from build123d import *

# Parameters (mm, degrees)
EXTRUDE_4_OUTLINE_R  = 1.5999968
EXTRUDE_4_OUTLINE_W  = 44.323
EXTRUDE_4_OUTLINE_H  = 54.229
EXTRUDE_4_DEPTH      = 1.5
EXTRUDE_5_DEPTH      = 1.5
EXTRUDE_5_DEPTH_BACK = 13
SKETCH_3_W           = 44.323
SKETCH_3_H           = 54.229
SKETCH_5_R           = 1.27
SKETCH_5_W           = 14.0000228
SKETCH_5_H           = 32.0000376
EXTRUDE_6_DEPTH      = 13
EXTRUDE_8_DEPTH      = 1.5
EXTRUDE_8_DEPTH_BACK = 20
SKETCH_6_W           = 38.989
SKETCH_6_H           = 65.9999442
SKETCH_6_R           = 1.016
SKETCH_6_R_2         = 0.4572


# Read off the part's stored shape, not the designer's step: the extrude step
with BuildPart() as part:
    # Extrude 4 outline → Extrude 4 (new body)
    with BuildSketch(Plane.XY):
        with BuildLine():
            ThreePointArc((122.299984025, 9.019649552), (120.835516371, 12.55516818), (117.299994025, 14.019626857))
            Line((117.299994025, 14.019626857), (4.999990016, 14.019626857))
            ThreePointArc((4.999990016, 14.019626857), (1.464472156, 12.555172669), (1.1e-08, 9.019662248))
            Line((1.1e-08, 9.019662248), (1.1e-08, -60.980388257))
            ThreePointArc((1.1e-08, -60.980388257), (1.464467665, -64.515906885), (4.999990011, -65.980365562))
            Line((4.999990011, -65.980365562), (117.29999402, -65.980365562))
            ThreePointArc((117.29999402, -65.980365562), (120.835516369, -64.515906884), (122.299984025, -60.980388255))
            Line((122.299984025, -60.980388255), (122.299984025, 9.019649552))
        make_face()
        with Locations((4.999990011, -53.480365152)):
            Circle(EXTRUDE_4_OUTLINE_R, mode=Mode.SUBTRACT)
        with Locations((117.299994011, -53.480365152)):
            Circle(EXTRUDE_4_OUTLINE_R, mode=Mode.SUBTRACT)
        Polygon((11.635994011, 6.209634848), (15.826994011, 6.209634848), (15.826994011, 10.273634848), (17.183354011, 11.797634848), (45.290994011, 11.797634848), (46.306994011, 10.781634848), (46.306994011, 6.209634848), (50.624994011, 6.209634848), (50.624994011, -59.790309352), (11.635994011, -59.790309352), align=None, mode=Mode.SUBTRACT)
        with Locations((4.999990011, 1.519524848)):
            Circle(EXTRUDE_4_OUTLINE_R, mode=Mode.SUBTRACT)
        with Locations((74.818494011, -20.269865152)):
            Rectangle(EXTRUDE_4_OUTLINE_W, EXTRUDE_4_OUTLINE_H, mode=Mode.SUBTRACT)
        with Locations((117.299994011, 1.519524848)):
            Circle(EXTRUDE_4_OUTLINE_R, mode=Mode.SUBTRACT)
    extrude(amount=EXTRUDE_4_DEPTH)



with BuildPart() as body_2:
    # Sketch 3 → Extrude 5 (new, two sides: drawn at the far end of the back side and taken through both)
    with BuildSketch(Plane.XY.offset(-EXTRUDE_5_DEPTH_BACK)):
        with Locations((74.818494011, -20.269865152)):
            Rectangle(SKETCH_3_W, SKETCH_3_H)
    extrude(amount=EXTRUDE_5_DEPTH + EXTRUDE_5_DEPTH_BACK)


with BuildPart() as part_1:
    add(part.part)

    add(body_2.part)  # Extrude 6 merges body 2
    # Sketch 5 → Extrude 6 (add)
    # profile 1 of 3: a face of its own
    with BuildSketch(Plane.XY):
        Polygon((46.306994011, 6.209634848), (15.826994011, 6.209634848), (15.826994011, -42.812365152), (17.096994011, -44.082365152), (27.256994011, -44.082365152), (27.256994011, -44.590365152), (34.876994011, -44.590365152), (34.876994011, -44.082365152), (45.036994011, -44.082365152), (46.306994011, -42.812365152), align=None)
        with Locations(Location((18.366994011, -41.542365152, 0), (0, 0, 180))):
            Circle(SKETCH_5_R, mode=Mode.SUBTRACT)
        with Locations(Location((43.766994011, -41.542365152, 0), (0, 0, 180))):
            Circle(SKETCH_5_R, mode=Mode.SUBTRACT)
    # profile 2 of 3: a face of its own
    with BuildSketch(Plane.XY):
        Polygon((15.826994011, 10.273634848), (15.826994011, 6.209634848), (46.306994011, 6.209634848), (46.306994011, 10.781634848), (45.290994011, 11.797634848), (38.686994011, 11.797634848), (23.446994011, 11.797634848), (17.183354011, 11.797634848), align=None)
        with Locations(Location((18.366994011, 9.257634848, 0), (0, 0, 180))):
            Circle(SKETCH_5_R, mode=Mode.SUBTRACT)
        with Locations(Location((43.766994011, 9.257634848, 0), (0, 0, 180))):
            Circle(SKETCH_5_R, mode=Mode.SUBTRACT)
    # profile 3 of 3: a face of its own
    with BuildSketch(Plane.XY):
        with Locations((74.897005411, -13.257382352)):
            Rectangle(SKETCH_5_W, SKETCH_5_H)
    extrude(amount=EXTRUDE_6_DEPTH)

    # Sketch 6 → Extrude 8 (add, two sides: drawn at the far end of the back side and taken through both)
    with BuildSketch(Plane.XY.offset(-EXTRUDE_8_DEPTH_BACK)):
        with Locations((31.130494011, -26.790337252)):
            Rectangle(SKETCH_6_W, SKETCH_6_H)
        with Locations((14.556994011, -56.909365152)):
            Circle(SKETCH_6_R, mode=Mode.SUBTRACT)
        with Locations((23.700994011, -57.290365152)):
            Circle(SKETCH_6_R_2, mode=Mode.SUBTRACT)
        with Locations((38.940994011, -57.290365152)):
            Circle(SKETCH_6_R_2, mode=Mode.SUBTRACT)
        with Locations((47.957994011, -56.909365152)):
            Circle(SKETCH_6_R, mode=Mode.SUBTRACT)
    extrude(amount=EXTRUDE_8_DEPTH + EXTRUDE_8_DEPTH_BACK)


solid = part_1.part
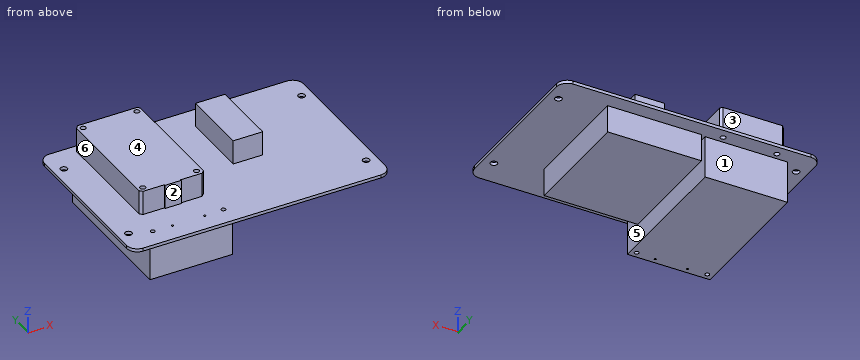
Could you check a few things on this model? Use its own coordinates, in mm. Face numbers are marked on the shaded views. A direction names the side the tool comes from. Coordinates: 2 decimals unless noted, no trailing zeros. Order: outer loops, then holes, each group sorted by start corner. A loop starts at its lowest first (then second) coordinate and runs counter-clockwise, first axis right, second up.
Q1. Thinking about a two-plate mould opening in X: for the marked faces 4, 5 and 6, which applies, released by +X, released by -X, zero draft, split by the parting line, or undercut?
Q2. Which directions (+Z, -Z, +X, -X, +Y, -Y) give clear straight access to the entire face, cutting with the end or side of a thin tool? Please do the marked faces 1, 2 and 3.
Q3. Will these pins go through, and if not, where does the flat tip stop? pin 1 (1.5 mm diameter, centred on y = -14.5, z = 7, fed in from -X); pin 2 (8 mm diameter, centred on x = 27.5, z = -4.5, fed in from +Y); pin 3 (5 mm diameter, centred on y = -20, z = -14, fed in from +X); pin 4 (12.5 mm diameter, centred on x = 73, z = 7, fed in from +Y).
Q4. Please list where these lines run through material, in increasing order: L1, parallel to X at y = -8, z = 9.5; L2, parallel to X at y = -32.5, z = -2 (3 decimals); L3, parallel to Z at x = 67, y = -2.5.
Q5. Suppose I cut it at B-B on y = -17.5. Please give me the cut outline in (x, z) (3 decimals).
Q6. Suppose I cut it at C-C on z = -17. Please give me the cut outline in (x, y) (3 decimals), and give its area (3 significant figures).
Q7. Suppose I cut it at A-A on z = 11.5. Please give me the cut outline in (x, y).
Q8. Suppose I cut it at D-D on x = 87. Please give me the cut outline in (y, z).
Answer:
1. face 4: zero draft
1. face 5: undercut
1. face 6: released by -X
2. face 1: -Z, -X, +Y
2. face 2: +Z, +X, -X, -Y
2. face 3: +Z, +X, -X, +Y
3. pin 1: stops at x = 15.83
3. pin 2: stops at y = 6.21
3. pin 3: stops at x = 96.98
3. pin 4: stops at y = 14.02
4. L1: x = 15.83 to 46.31, 67.9 to 81.9
4. L2: x = 11.636 to 50.625, 52.657 to 96.98
4. L3: z = -13 to 1.5
5. outline: (0, 0) - (11.636, 0) - (11.636, -20) - (50.625, -20) - (50.625, 0) - (52.657, 0) - (52.657, -13) - (96.98, -13) - (96.98, 0) - (122.3, 0) - (122.3, 1.5) - (81.897, 1.5) - (81.897, 13) - (67.897, 13) - (67.897, 1.5) - (46.307, 1.5) - (46.307, 13) - (15.827, 13) - (15.827, 1.5) - (0, 1.5) - close
6. outline: (11.636, -59.79) - (50.625, -59.79) - (50.625, 6.21) - (11.636, 6.21) - close; hole circle Ø2.032 at (14.557, -56.909); hole circle Ø0.914 at (23.701, -57.29); hole circle Ø0.914 at (38.941, -57.29); hole circle Ø2.032 at (47.958, -56.909)
6. area: 2,570 mm2
7. outline: (15.83, -42.81) - (17.1, -44.08) - (27.26, -44.08) - (27.26, -44.59) - (34.88, -44.59) - (34.88, -44.08) - (45.04, -44.08) - (46.31, -42.81) - (46.31, 10.78) - (45.29, 11.8) - (17.18, 11.8) - (15.83, 10.27) - close; (67.9, -29.26) - (81.9, -29.26) - (81.9, 2.74) - (67.9, 2.74) - close; hole circle Ø2.54 at (18.37, -41.54); hole circle Ø2.54 at (18.37, 9.26); hole circle Ø2.54 at (43.77, -41.54); hole circle Ø2.54 at (43.77, 9.26)
8. outline: (-65.98, 0) - (-47.38, 0) - (-47.38, -13) - (6.84, -13) - (6.84, 0) - (14.02, 0) - (14.02, 1.5) - (-65.98, 1.5) - close
